CAD build for the part. Positions are in the model's coordinates, mm. Face numbers are marked on the shaded views. A direction names the side the tool comes from. Give positions to 0.01 mm unless a question says otherwise; leave off trailing zeros. Order: outer loops, then holes, each group sorted by start corner. A loop starts at its lowest first (then second) coordinate and runs counter-clockwise, first axis right, second up. Notation, with made-up numbers: M 85,2.5 L 140,2.5 A20 ccw 140,40.5 Z; hole C -5.5,67 d5. An arc over 180 degrees is marked long. Put each result on its own line as item: value. Start each with the question number.
1) Cut at A-A (y = 0). Write the cut outline in (x, z).
2) Drill centre lines: line 1 (Y direction, x = -35.5, z = 10); line 2 (X direction, y = -13, z = 3.5); line 3 (X direction, y = 6, z = 7.25). Where is each one in solid material? Low to high. Write a range as [from, to].
3) Cut at C-C (z = 17.25). Write the cut outline in (x, y).
4) Cut at D-D (y = 20). Write the cut outline in (x, z).
5) Pin check, flat tips, straight feed: pin 1 (12 mm diameter, centred on x = 28, z = 11.5, fed in from +Y); pin 2 (10 mm diameter, centred on x = -6, y = 4.5, fed in from -Z); pin 3 (1 mm diameter, centred on y = -4.5, z = 11.5, fed in from +X); pin 4 (7.5 mm diameter, centred on x = 47.5, z = 16.5, fed in from +Y). Stop position of each tip, or through.
6) Two-plate mould, pull along X, no slides. Class the marked faces 4, 5, 6 and 7: released by +X, released by -X, zero draft, split by the parting line, or undercut.
7) Tool access for the marked faces 1, 2 and 3: list every direction of +Z, -Z, +X, -X, +Y, -Y with a clear straight run to the whole face (end or side of a thin tool).
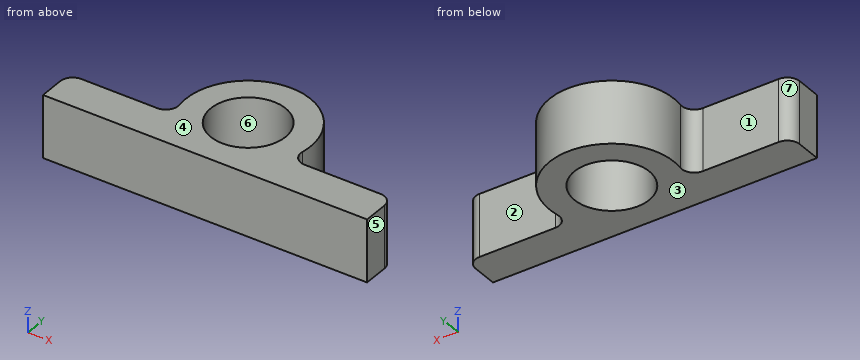
```python
from build123d import *

# Parameters (mm, degrees)
SKETCH1_R           = 15
BOSS_EXTRUDE1_DEPTH = 25


with BuildPart() as part:
    # Sketch1 → Boss-Extrude1 (new body)
    with BuildSketch(Plane.XY):
        with BuildLine():
            Line((-65, -25), (-65, -15))
            ThreePointArc((-65, -15), (-63.535533906, -11.464466094), (-60, -10))
            Line((-60, -10), (-29.580398915, -10))
            ThreePointArc((-29.580398915, -10), (-25.761585836, -8.227486122), (-24.65033243, -4.166666667))
            ThreePointArc((-24.65033243, -4.166666667), (0, 25), (24.65033243, -4.166666667))
            ThreePointArc((24.65033243, -4.166666667), (25.761585836, -8.227486122), (29.580398915, -10))
            Line((29.580398915, -10), (60, -10))
            ThreePointArc((60, -10), (63.535533906, -11.464466094), (65, -15))
            Line((65, -15), (65, -25))
            Line((65, -25), (-65, -25))
        make_face()
        Circle(SKETCH1_R, mode=Mode.SUBTRACT)
    extrude(amount=BOSS_EXTRUDE1_DEPTH)


solid = part.part
```
Solution:
1. outline: M -25,0 L -15,0 L -15,25 L -25,25 Z; M 15,0 L 25,0 L 25,25 L 15,25 Z
2. line 1: [-25, -10]
2. line 2: [-64.58, -7.48], [7.48, 64.58]
2. line 3: [-24.27, -13.75], [13.75, 24.27]
3. outline: M -65,-25 L 65,-25 L 65,-15 A5 ccw 60,-10 L 29.58,-10 A5 cw 24.65,-4.17 A25 ccw long -24.65,-4.17 A5 cw -29.58,-10 L -60,-10 A5 ccw -65,-15 Z; hole C 0,0 d30
4. outline: M -15,0 L 15,0 L 15,25 L -15,25 Z
5. pin 1: y = 11.87
5. pin 2: through
5. pin 3: x = 24.68
5. pin 4: y = -10
6. face 4: zero draft
6. face 5: released by +X
6. face 6: undercut
6. face 7: released by -X
7. face 1: +Z, -Z, -X, +Y
7. face 2: +Z, -Z, +X, +Y
7. face 3: -Z, +X, -X, +Y, -Y
